Autodesk Inventor part; units mm, degrees
ref_plane "РабПлоскость1" through (19.6828, -0.4261, 0) normal (0, 0, 1) x (0.9982449, -0.0592218, 0)
ref_plane "YZ Plane" through (0, 0, 0) normal (1, 0, 0) x (0, 1, 0)
ref_plane "XY Plane" through (0, 0, 0) normal (0, 0, 1) x (1, 0, 0)
ref_plane "РабПлоскость1" through (19.6828, -0.4261, 0) normal (0, 0, 1) x (0.9982449, -0.0592218, 0)
sketch "Эскиз1" plane through (19.6828, -0.4261, 0) normal (0, 0, 1) x (0.9982449, -0.0592218, 0)
  circle A0 centre (-7.1954, 0) radius 10
  circle A1 centre (-7.1954, 0) radius 12.5
  point P0 (-19.6734, -0.7403)
  point P1 (0.3275, 9.9828)
  point P2 (1.4551, -9.0233)
  point P3 (-15.8459, 9.0233)
  point P4 (-14.7183, -9.9828)
extrude "Выдавливание1" add sketch "Эскиз1" against normal blind 11.75 contours A0
sketch "Эскиз2" plane through (12.5, 0, 0) normal (0, 0, 1) x (1, 0, 0)
  circle A0 centre (0, 0) radius 12.5
  point P0 (-12.5, 0)
extrude "Выдавливание2" add sketch "Эскиз2" along normal blind 3
chamfer "Фаска1" distance 0.5 angle 45 1 edges at (0, 0, 3)
sketch "Эскиз8" plane through (12.5, 0, -11.75) normal (0, 0, -1) x (-1, 0, 0)
  circle A0 centre (0, 0) radius 6
  point P0 (12.5, 0)
  dimension "d23" = 12
extrude "Выдавливание8" cut sketch "Эскиз8" against normal blind 5
sketch "Эскиз9" plane through (12.5, 0, -6.75) normal (0, 0, -1) x (-1, 0, 0)
  circle A0 centre (0, 0) radius 4.15
  circle A1 centre (0, 0) radius 6
  point P0 (12.5, 0)
  dimension "d26" = 8.3
extrude "Выдавливание9" cut sketch "Эскиз9" against normal through all contours A0
ref_plane "РабПлоскость3" through (12.5, 10, 0) normal (0, 1, 0) x (-1, 0, 0)
sketch "Эскиз12" plane through (12.5, 0, -11.75) normal (0, 0, -1) x (-1, 0, 0)
  circle A0 centre (0, 0) radius 9.6
  circle A1 centre (0, 0) radius 10
  point P0 (12.5, 0)
  dimension "d35" = 19.2
  dimension "d36" = 20
extrude "Выдавливание12" cut sketch "Эскиз12" against normal up to surface (11.75 mm away)
properties part number "bushing"
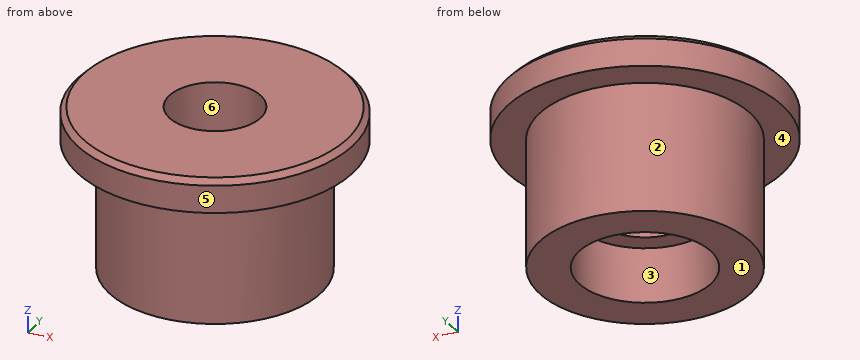
The listing builds one solid part. Answer for the finished solid, in the listing's coordinates (mm). Face numbers are marked on the shaded views. A direction names the side the tool comes from. Give positions to 0.01 mm unless a question says otherwise; leave off trailing zeros. Order: outer loops, then holes, each group sorted by start corner. A loop starts at its lowest first (then second) coordinate and runs counter-clockwise, first axis right, second up. Notation, with made-up numbers: (-14, 48.25) -> (15, 48.25) arc R30 ccw to (15, 80.25) -> close; hole circle Ø10 at (80.25, -40). An arc over 180 degrees is marked (long way). Answer as a JSON object with one key per item and string values. Group by question number.
Item 1: The part is cut by section C-C on z = -1. Write down the section's boundary in (x, y), and give its area (3 significant figures).
Item 2: A tool of negligible diameter and unlimited length cuts with its end or side. For the marked faces 1 and 2, from which of +Z, -Z, +X, -X, +Y, -Y can it reach the whole face along a straight path? Write none if from no direction.
Item 3: Consider L1, parallel to Y at x = 12.5, z = -10.3; L2, parallel to X at y = 0.25, z = 1.5; L3, parallel to Z at x = 8.5, y = -1.25. Determine where each line is inside the solid, lowest interval first. Write a range as from..to.
Item 4: The part is cut by section B-B on y = 0. Write down the section's boundary in (x, z), and give its area (3 significant figures).
Item 5: The part is cut by section A-A on x = 12.5. Write down the section's boundary in (y, z).
Item 6: Determine the mould class of the marked faces 3, 4, 5 and 6 for opening direction X: pulls with the +X half, pulls with the -X half, needs draft (parallel to the pull), parting line crosses it, or undercut.
Item 7: Flat-ended cylindrical pins translate along their axes: pin 1 (9.5 mm diameter, centred on x = 12.5, y = 0, fed in from -Z); pin 2 (4 mm diameter, centred on y = -7, z = -7.5, fed in from +X); pin 3 (7.5 mm diameter, centred on x = 12.5, y = 0, fed in from +Z); pin 4 (3 mm diameter, centred on x = 14.5, z = -5.5, fed in from -Y). Find the tip coordinate at first contact, or state that the pin passes through.
Result set:
{
 "1": {"outline": "circle Ø19.2 at (12.5, 0); hole circle Ø8.3 at (12.5, 0)", "area": "235 mm²"},
 "2": {"face 1": "-Z, +X, -X, +Y, -Y", "face 2": "-Z"},
 "3": {"L1": "-9.6..-6, 6..9.6", "L2": "0..8.36, 16.64..25", "L3": "-6.75..3"},
 "4": {"outline": "(0, 0) -> (2.9, 0) -> (2.9, -11.75) -> (6.5, -11.75) -> (6.5, -6.75) -> (8.35, -6.75) -> (8.35, 3) -> (0.5, 3) -> (0, 2.5) -> close; (16.65, -6.75) -> (18.5, -6.75) -> (18.5, -11.75) -> (22.1, -11.75) -> (22.1, 0) -> (25, 0) -> (25, 2.5) -> (24.5, 3) -> (16.65, 3) -> close", "area": "159 mm²"},
 "5": {"outline": "(-12.5, 0) -> (-9.6, 0) -> (-9.6, -11.75) -> (-6, -11.75) -> (-6, -6.75) -> (-4.15, -6.75) -> (-4.15, 3) -> (-12, 3) -> (-12.5, 2.5) -> close; (4.15, -6.75) -> (6, -6.75) -> (6, -11.75) -> (9.6, -11.75) -> (9.6, 0) -> (12.5, 0) -> (12.5, 2.5) -> (12, 3) -> (4.15, 3) -> close"},
 "6": {"face 3": "undercut", "face 4": "needs draft", "face 5": "parting line crosses it", "face 6": "undercut"},
 "7": {"pin 1": "z = -6.75", "pin 2": "x = 20.7", "pin 3": "through", "pin 4": "y = -9.59"}
}
